CAD build for the part. Positions are in the model's coordinates, mm. A direction names the side the tool comes from. Give positions to 0.01 mm unless a question says otherwise; leave off trailing zeros. Write each loop counter-clockwise with the first axis right and the second up, starting at its lowest first coordinate (ties: lowest second). Pieces come first, ordered by that corner, then holes. Notation, with made-up numbers: (-32.5, 51.25) -> (25.5, 51.25) arc R13 ccw to (25.5, 63.25) -> close; hole circle Ø11 at (-18, -38). An arc over 180 degrees is marked (long way). Answer as a JSON object with one key per item and string values.
```python
from build123d import *

# Parameters (mm, degrees)
BOSS_EXTRUDE1_DEPTH = 1
FILLET1_R           = 2
FILLET2_R           = 1


with BuildPart() as part:
    # Sketch1 → Boss-Extrude1 (new body)
    with BuildSketch(Plane.XY):
        with BuildLine():
            Line((-9, 6), (9, 6))
            ThreePointArc((9, 6), (9.707106781, 5.707106781), (10, 5))
            Line((10, 5), (10, -5))
            ThreePointArc((10, -5), (9.707106781, -5.707106781), (9, -6))
            Line((9, -6), (-9, -6))
            ThreePointArc((-9, -6), (-9.707106781, -5.707106781), (-10, -5))
            Line((-10, -5), (-10, 5))
            ThreePointArc((-10, 5), (-9.707106781, 5.707106781), (-9, 6))
        make_face()
    extrude(amount=BOSS_EXTRUDE1_DEPTH)

    # Sketch2 → Revolve2 (revolve)
    with BuildSketch(Plane(origin=(0, 0, 0), x_dir=(1, 0, 0), z_dir=(0, 1, 0))):
        with BuildLine():
            Line((0, -1), (0, -54))
            Line((0, -54), (12.5, -54))
            ThreePointArc((12.5, -54), (6.778694886, -52.527781041), (1, -51.3))
            Line((1, -51.3), (1, -1))
            Line((1, -1), (0, -1))
        make_face()
    revolve(axis=Axis((0, 0, 1), (0, 0, 1)))

    # Fillet1
    fillet1_edges = [part.edges().sort_by_distance(p)[0] for p in [
        (-1, 0, 51.3),
    ]]
    fillet(fillet1_edges, radius=FILLET1_R)

    # Fillet2
    fillet2_edges = [part.edges().sort_by_distance(p)[0] for p in [
        (-1, 0, 1),
    ]]
    fillet(fillet2_edges, radius=FILLET2_R)


solid = part.part
```
1) Wall check: probe 1 along Z at (x, y) = (-2.75, 0.75); probe 2 along Y at (x, z) = (0, 33); probe 3 along Z at (x, y) = (0, 4.5). Give the ranges that are in metal, low to high.
Model answer:
{"probe 1": "z = 0 to 1, 51.67 to 54", "probe 2": "y = -1 to 1", "probe 3": "z = 0 to 1, 52.01 to 54"}
2) Slice it at A-A (z = 5). List the corners of the cut face in (x, y).
Model answer:
{"outline": "circle Ø2 at (0, 0)"}
3) Pin check, flat tips, straight feed: pin 1 (12 mm diameter, centred on y = 3, z = 41, fed in from +X); pin 2 (0.8 mm diameter, centred on y = 2, z = 0.5, fed in from -X); pin 3 (0.8 mm diameter, centred on x = -4, z = 0.5, fed in from +Y). Stop position of each tip, or through.
Model answer:
{"pin 1": "stops at x = 1", "pin 2": "stops at x = -10", "pin 3": "stops at y = 6"}
4) 3-axis set-ups, long thin cutter, end or side, ignore diameter. For faces 5 (the flat face through (10, 0.1, 0.5)), 6 (the cylindrical face through (-9.715, 5.699, 0.493)), 7 (the flat face through (0.1, -6, 0.5)), 8 (the cylindrical face through (9.715, -5.699, 0.493)), 9 (the cylindrical face through (-9.699, -5.715, 0.493)): which of +Z, -Z, +X, -X, +Y, -Y reach the whole face in a straight line?
Model answer:
{"face 5": "-Z, +X, +Y, -Y", "face 6": "-Z, -X, +Y", "face 7": "-Z, +X, -X, -Y", "face 8": "-Z, +X, -Y", "face 9": "-Z, -X, -Y"}
5) Mould opens along Z. For faces 1 (the flat face through (0, 0, 54)), 2 (the flat face through (2.4, 0.1, 1)), 3 (the cylindrical face through (9.699, 5.715, 0.493)), 4 (the cylindrical face through (1, 0, 25)) say: released by +Z, released by -Z, zero draft, split by the parting line, or undercut.
Model answer:
{"face 1": "released by +Z", "face 2": "undercut", "face 3": "zero draft", "face 4": "undercut"}
